from build123d import *

# Parameters (mm, degrees)
BOSS_EXTRUDE1_DEPTH      = 8.45
SKETCH2_W                = 12
SKETCH2_H                = 30
CUT_EXTRUDE1_DEPTH       = 8.45
CUT_EXTRUDE2_DEPTH       = 8.45
SKETCH4_W                = 0.8
SKETCH4_H                = 1.9
CUT_EXTRUDE3_DEPTH       = 8.45
SKETCH5_W                = 0.8
SKETCH5_H                = 1.9
CUT_EXTRUDE4_DEPTH       = 8.45
BOSS_EXTRUDE2_DEPTH      = 2.5
CUT_EXTRUDE5_DEPTH       = 3
CUT_EXTRUDE5_DEPTH_BACK  = 3
CUT_EXTRUDE6_DEPTH       = 5
CUT_EXTRUDE6_DEPTH_BACK  = 5
SKETCH9_W                = 8.3
SKETCH9_H                = 18.5
CUT_EXTRUDE7_DEPTH       = 3
BOSS_EXTRUDE3_DEPTH      = 3.6
BOSS_EXTRUDE3_DEPTH_BACK = 3.6
SKETCH11_W               = 3
SKETCH11_H               = 4.5
CUT_EXTRUDE8_DEPTH       = 30
BOSS_EXTRUDE4_DEPTH      = 1.85
CUT_EXTRUDE9_DEPTH       = 30
CUT_EXTRUDE10_DEPTH      = 0.85


with BuildPart() as part:
    # Sketch1 → Boss-Extrude1 (new body)
    with BuildSketch(Plane(origin=(0, 0, 0), x_dir=(0, 0, -1), z_dir=(1, 0, 0))):
        with BuildLine():
            Line((-4.2, 0), (4.2, 0))
            ThreePointArc((4.2, 0), (4.694974747, 0.205025253), (4.9, 0.7))
            Line((4.9, 0.7), (4.9, 27.316294728))
            ThreePointArc((4.9, 27.316294728), (4.803647153, 27.611369254), (4.551724095, 27.792718697))
            ThreePointArc((4.551724095, 27.792718697), (-2.2e-08, 28.5), (-4.551724138, 27.792718684))
            ThreePointArc((-4.551724138, 27.792718684), (-4.803647166, 27.611369236), (-4.9, 27.316294728))
            Line((-4.9, 27.316294728), (-4.9, 0.7))
            ThreePointArc((-4.9, 0.7), (-4.694974747, 0.205025253), (-4.2, 0))
        make_face()
    extrude(amount=BOSS_EXTRUDE1_DEPTH)

    # Sketch2 → Cut-Extrude1 (cut)
    with BuildSketch(Plane(origin=(4.7, 0, 0), x_dir=(0, 0, -1), z_dir=(1, 0, 0))):
        with Locations((0, 14)):
            Rectangle(SKETCH2_W, SKETCH2_H)
        with BuildLine():
            Line((-4.15, 6.25), (-4.15, 0.95))
            ThreePointArc((-4.15, 0.95), (-4.091421356, 0.808578644), (-3.95, 0.75))
            Line((-3.95, 0.75), (3.95, 0.75))
            ThreePointArc((3.95, 0.75), (4.091421356, 0.808578644), (4.15, 0.95))
            Line((4.15, 0.95), (4.15, 6.25))
            ThreePointArc((4.15, 6.25), (4.091421356, 6.391421356), (3.95, 6.45))
            Line((3.95, 6.45), (-3.95, 6.45))
            ThreePointArc((-3.95, 6.45), (-4.091421356, 6.391421356), (-4.15, 6.25))
        make_face(mode=Mode.SUBTRACT)
    extrude(amount=CUT_EXTRUDE1_DEPTH, mode=Mode.SUBTRACT)

    # Sketch3 → Cut-Extrude2 (cut)
    with BuildSketch(Plane(origin=(4.7, 0, 0), x_dir=(0, 0, -1), z_dir=(1, 0, 0))):
        with BuildLine():
            Line((-3.45, 5.55), (-3.45, 1.65))
            ThreePointArc((-3.45, 1.65), (-3.391421356, 1.508578644), (-3.25, 1.45))
            Line((-3.25, 1.45), (-1.05, 1.45))
            Line((-1.05, 1.45), (-1.05, 2.25))
            Line((-1.05, 2.25), (-0.75, 2.25))
            Line((-0.75, 2.25), (-0.75, 1.45))
            Line((-0.75, 1.45), (0.75, 1.45))
            Line((0.75, 1.45), (0.75, 2.25))
            Line((0.75, 2.25), (1.05, 2.25))
            Line((1.05, 2.25), (1.05, 1.45))
            Line((1.05, 1.45), (3.25, 1.45))
            ThreePointArc((3.25, 1.45), (3.391421356, 1.508578644), (3.45, 1.65))
            Line((3.45, 1.65), (3.45, 5.55))
            ThreePointArc((3.45, 5.55), (3.391421356, 5.691421356), (3.25, 5.75))
            Line((3.25, 5.75), (-3.25, 5.75))
            ThreePointArc((-3.25, 5.75), (-3.391421356, 5.691421356), (-3.45, 5.55))
        make_face()
    extrude(amount=CUT_EXTRUDE2_DEPTH, mode=Mode.SUBTRACT)

    # Sketch4 → Cut-Extrude3 (cut)
    with BuildSketch(Plane(origin=(4.7, 0, 0), x_dir=(0, 0, -1), z_dir=(1, 0, 0))):
        with Locations((2, 4.1)):
            Rectangle(SKETCH4_W, SKETCH4_H)
    extrude(amount=-CUT_EXTRUDE3_DEPTH, mode=Mode.SUBTRACT)

    # Sketch5 → Cut-Extrude4 (cut)
    with BuildSketch(Plane(origin=(4.7, 0, 0), x_dir=(0, 0, -1), z_dir=(1, 0, 0))):
        with Locations((-2, 4.1)):
            Rectangle(SKETCH5_W, SKETCH5_H)
    extrude(amount=-CUT_EXTRUDE4_DEPTH, mode=Mode.SUBTRACT)

    # Sketch6 → Boss-Extrude2 (add)
    with BuildSketch(Plane(origin=(4.7, 0, 0), x_dir=(0, 0, -1), z_dir=(1, 0, 0))):
        with BuildLine():
            Line((-2.5, 20.341875815), (-2.5, 10.775))
            Line((-2.5, 10.775), (2.5, 10.775))
            Line((2.5, 10.775), (2.5, 20.341875815))
            ThreePointArc((2.5, 20.341875815), (2.454337374, 20.50097484), (2.33125, 20.611641338))
            ThreePointArc((2.33125, 20.611641338), (1.469638379, 21.38630682), (1.15, 22.5))
            Line((1.15, 22.5), (1.15, 28.175404594))
            ThreePointArc((1.15, 28.175404594), (1.068178929, 28.381312231), (0.867346966, 28.474902645))
            ThreePointArc((0.867346966, 28.474902645), (1.4e-08, 28.5), (-0.867346939, 28.474902647))
            ThreePointArc((-0.867346939, 28.474902647), (-1.068178919, 28.381312241), (-1.15, 28.175404594))
            Line((-1.15, 28.175404594), (-1.15, 22.5))
            ThreePointArc((-1.15, 22.5), (-1.469638379, 21.38630682), (-2.33125, 20.611641338))
            ThreePointArc((-2.33125, 20.611641338), (-2.454337374, 20.50097484), (-2.5, 20.341875815))
        make_face()
    extrude(amount=BOSS_EXTRUDE2_DEPTH)

    # Sketch7 → Cut-Extrude5 (cut, two sides)
    with BuildSketch(Plane.XY) as cut_extrude5_sk:
        Polygon((4.7, 10.775), (12.2, 10.775), (12.2, 30.775), (7.2, 30.775), (7.2, 26.65), (6.95, 26.4), (6.95, 24.25), (6.2, 23.5), (6.2, 12.275), align=None)
    extrude(amount=CUT_EXTRUDE5_DEPTH, mode=Mode.SUBTRACT)
    extrude(cut_extrude5_sk.sketch, amount=-CUT_EXTRUDE5_DEPTH_BACK, mode=Mode.SUBTRACT)

    # Sketch8 → Cut-Extrude6 (cut, two sides)
    with BuildSketch(Plane(origin=(4.7, 0, 0), x_dir=(0, 0, -1), z_dir=(1, 0, 0))) as cut_extrude6_sk:
        with BuildLine():
            Line((-7, 20.4), (-3.25, 20.4))
            ThreePointArc((-3.25, 20.4), (-1.15, 22.5), (-3.25, 24.6))
            Line((-3.25, 24.6), (-6, 24.6))
            Line((-6, 24.6), (-6, 30.06))
            Line((-6, 30.06), (-4.15, 30.06))
            Line((-4.15, 30.06), (-4.15, 27.06))
            Line((-4.15, 27.06), (-1.6, 27.06))
            Line((-1.6, 27.06), (-1.6, 29.06))
            Line((-1.6, 29.06), (1.6, 29.06))
            Line((1.6, 29.06), (1.6, 27.06))
            Line((1.6, 27.06), (4.15, 27.06))
            Line((4.15, 27.06), (4.15, 30.06))
            Line((4.15, 30.06), (6, 30.06))
            Line((6, 30.06), (6, 24.6))
            Line((6, 24.6), (3.25, 24.6))
            ThreePointArc((3.25, 24.6), (1.15, 22.5), (3.25, 20.4))
            Line((3.25, 20.4), (7, 20.4))
            Line((7, 20.4), (7, 31.06))
            Line((7, 31.06), (-7, 31.06))
            Line((-7, 31.06), (-7, 20.4))
        make_face()
    extrude(amount=CUT_EXTRUDE6_DEPTH, mode=Mode.SUBTRACT)
    extrude(cut_extrude6_sk.sketch, amount=-CUT_EXTRUDE6_DEPTH_BACK, mode=Mode.SUBTRACT)

    # Sketch9 → Cut-Extrude7 (cut)
    with BuildSketch(Plane(origin=(0, 0, 0), x_dir=(0, 0, -1), z_dir=(1, 0, 0))):
        with Locations((0, 10)):
            Rectangle(SKETCH9_W, SKETCH9_H)
    extrude(amount=CUT_EXTRUDE7_DEPTH, mode=Mode.SUBTRACT)

    # Sketch10 → Boss-Extrude3 (add, two sides)
    with BuildSketch(Plane.XY) as boss_extrude3_sk:
        with BuildLine():
            Line((-1.97, 27.06), (-1.97, 26.31))
            Line((-1.97, 26.31), (0, 26.31))
            Line((0, 26.31), (0, 27.06))
            Line((0, 27.06), (-1.0486903, 27.06))
            ThreePointArc((-1.0486903, 27.06), (-1.125852758, 27.096392178), (-1.146853018, 27.1790809))
            Line((-1.146853018, 27.1790809), (-1.035788259, 27.75045955))
            ThreePointArc((-1.035788259, 27.75045955), (-1.046288389, 27.791803911), (-1.084869618, 27.81))
            Line((-1.084869618, 27.81), (-1.323188014, 27.81))
            ThreePointArc((-1.323188014, 27.81), (-1.413986114, 27.788201305), (-1.484991413, 27.72755705))
            Line((-1.484991413, 27.72755705), (-1.97, 27.06))
        make_face()
    extrude(amount=BOSS_EXTRUDE3_DEPTH)
    extrude(boss_extrude3_sk.sketch, amount=-BOSS_EXTRUDE3_DEPTH_BACK)

    # Sketch11 → Cut-Extrude8 (cut)
    with BuildSketch(Plane(origin=(0, 0, 0), x_dir=(1, 0, 0), z_dir=(0, 1, 0))):
        with Locations((-1.5, 0)):
            Rectangle(SKETCH11_W, SKETCH11_H)
    extrude(amount=CUT_EXTRUDE8_DEPTH, mode=Mode.SUBTRACT)

    # Sketch12 → Boss-Extrude4 (add)
    with BuildSketch(Plane(origin=(0, 0, 0), x_dir=(0, 0, -1), z_dir=(1, 0, 0))):
        with BuildLine():
            Line((-0.875, 28.474457419), (-0.875, 27.723110595))
            ThreePointArc((-0.875, 27.723110595), (0, 27.75), (0.875, 27.723110595))
            Line((0.875, 27.723110595), (0.875, 28.474457419))
            ThreePointArc((0.875, 28.474457419), (0, 28.5), (-0.875, 28.474457419))
        make_face()
    extrude(amount=-BOSS_EXTRUDE4_DEPTH)

    # Sketch13 → Cut-Extrude9 (cut)
    with BuildSketch(Plane(origin=(0, 0, 0), x_dir=(1, 0, 0), z_dir=(0, 1, 0))):
        Polygon((-3.85, -0.875), (-1.284314575, -0.875), (-1.85, -0.309314575), (-1.85, 0.309314575), (-1.284314575, 0.875), (-3.85, 0.875), align=None)
    extrude(amount=CUT_EXTRUDE9_DEPTH, mode=Mode.SUBTRACT)

    # Sketch14 → Cut-Extrude10 (cut)
    with BuildSketch(Plane(origin=(0, 0, 0), x_dir=(1, 0, 0), z_dir=(0, 1, 0))):
        with BuildLine():
            Line((1.1, 1.2), (1.1, -1.2))
            ThreePointArc((1.1, -1.2), (1.187867966, -1.412132034), (1.4, -1.5))
            Line((1.4, -1.5), (9.1, -1.5))
            Line((9.1, -1.5), (9.1, 1.5))
            Line((9.1, 1.5), (1.4, 1.5))
            ThreePointArc((1.4, 1.5), (1.187867966, 1.412132034), (1.1, 1.2))
        make_face()
    extrude(amount=CUT_EXTRUDE10_DEPTH, mode=Mode.SUBTRACT)


solid = part.part
Design review of the part built by this model. Coordinates are the model's own, in mm. A direction names the side the tool comes from. Coordinates: 2 decimals unless noted, no trailing zeros. Write each loop counter-clockwise with the first axis right and the second up, starting at its lowest first coordinate (ties: lowest second). Pieces come first, ordered by that corner, then holes. Notation, with made-up numbers: (13.25, -36.75) -> (38.25, -36.75) arc R18 ccw to (38.25, -11.75) -> close; hole circle Ø1 at (14, 75). An arc over 180 degrees is marked (long way). Write each question's results on one line, items separated by ' | '. Start each with the question number.
(1) Take a section at C-C on x = 5.25. Give the number of separate pieces and of enclosed holes in the cut face, and give its area (3 significant figures).
(2) For line 1 along Z through (x, y) = (1, 18); line 2 along Y through (x, z) = (3.5, 2); line 3 along Y through (x, z) = (6.25, 0.25), list the stretches that pass through material, from the lowest coordinate up. Write a range as from..to.
(3) Take a section at A-A on y = 15.75. Write out the cut boundary in (x, z).
(4) The part is to be moulded in two halves that separate along Y. For faces 1 (the face through (7, 4, 4.15)), 2 (the face through (4, 3.15, -2)), 3 (the face through (-1, 26.31, -3)), say which applies: pulls with the +Y half, pulls with the -Y half, needs draft (parallel to the pull), parting line crosses it, or undercut.
(5) Tool access review of faces 4 (the face through (6, 0.85, 0)), 5 (the face through (3, 10, 0)), 6 (the face through (7, 1.45, 2)), 7 (the face through (2, 24.6, -4)), 8 (the face through (3.4, 0.4, -1.5)): name each direction out of +Z, -Z, +X, -X, +Y, -Y from which nothing blocks a thin tool from reaching the whole face with its end or side.
(6) Clearance check with flat-ended pins moving along their axes: P1, Ø4, axis at x = 0, z = -2.5, coming from the +Y side; P2, Ø0.8, axis at x = -1, y = 27, coming from the -Z side; P3, Ø0.6, axis at x = 7, y = 1.5, coming from the +Z side. State where each tip first meets the part, or that it passes through.
Results found:
1) separate pieces: 2 | enclosed holes: 1 | area: 83.6 mm2
2) line 1: z = -4.9..-4.15, 4.15..4.9 | line 2: y = 0..3.15, 5.05..20.81, 24.19..27.06 | line 3: y = 0.85..1.45, 5.75..6.45, 23.55..28.5
3) outline: (0, -4.9) -> (4.7, -4.9) -> (4.7, -2.5) -> (6.2, -2.5) -> (6.2, 2.5) -> (4.7, 2.5) -> (4.7, 4.9) -> (0, 4.9) -> (0, 4.15) -> (3, 4.15) -> (3, -4.15) -> (0, -4.15) -> close
4) face 1: needs draft | face 2: undercut | face 3: pulls with the -Y half
5) face 4: +X, -X, -Y | face 5: -X | face 6: +X | face 7: -Z, +X, -X | face 8: +X, -Y
6) P1: stops at y = 28.49 | P2: stops at z = -3.6 | P3: stops at z = 4.15
